Autodesk Fusion 360 part; units mm, degrees
sketch "Sketch1" plane through (0, 0, 0) normal (0, 0, 1) x (1, 0, 0)
  line L0 (0, 0) -> (60, 0)
  line L1 (60, 0) -> (60, 60)
  line L2 (60, 60) -> (0, 60)
  line L3 (0, 60) -> (0, 0)
  line L4 (5, 5) -> (55, 5)
  line L5 (55, 5) -> (55, 55)
  line L6 (55, 55) -> (5, 55)
  line L7 (5, 55) -> (5, 5)
  dimension "d1" = 60
  dimension "d2" = 60
extrude "Extrude1" add sketch "Sketch1" along normal blind 50
extrude "Extrude2" add sketch "Sketch1" along normal blind 43 contours L4 L5 L6 L7
sketch "Sketch2" plane through (0, 0, 43) normal (0, 0, 1) x (-1, 0, 0)
  line L0 (-5, -55) -> (-5, -5)
  line L1 (-5, -5) -> (-55, -5)
  line L2 (-55, -5) -> (-55, -55)
  line L3 (-55, -55) -> (-5, -55)
  circle A0 centre (-15, -45) radius 5
  circle A1 centre (-30, -45) radius 5
  circle A2 centre (-45, -45) radius 5
  circle A3 centre (-15, -30) radius 5
  circle A4 centre (-30, -30) radius 5
  circle A5 centre (-45, -30) radius 5
  circle A6 centre (-15, -15) radius 5
  circle A7 centre (-30, -15) radius 5
  circle A8 centre (-45, -15) radius 5
  dimension "d7" = 10
  dimension "d8" = 10
  dimension "d9" = 10
  dimension "d10" = 10
  dimension "d11" = 10
  dimension "d12" = 10
  dimension "d13" = 10
  dimension "d14" = 10
  dimension "d15" = 10
hole "Hole1" at (45, 45, 43) at (45, 30, 43) at (45, 15, 43) at (30, 15, 43) at (30, 30, 43) at (30, 45, 43) at (15, 45, 43) at (15, 30, 43) at (15, 15, 43) direction (0, 0, -1) diameter 10 depth 2 tip angle 15
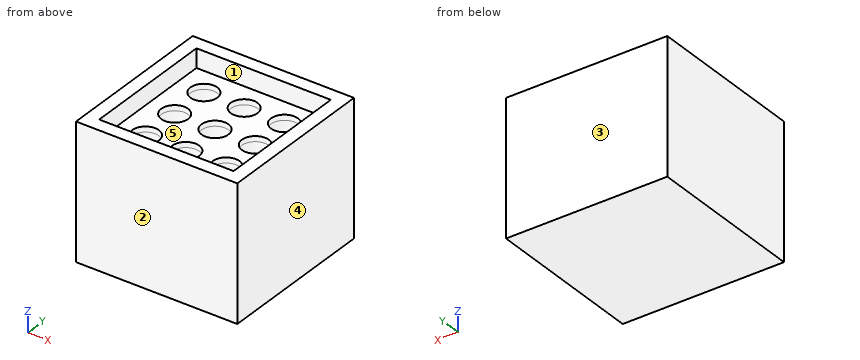
Geometry: final body of the model. Coordinates: model frame, mm. Face numbers are marked on the shaded views. A direction names the side the tool comes from. Round coordinates to 2 decimals unless told otherwise and drop trailing zeros. Loops run counter-clockwise (first coordinate to the right, second up) from the corner with the lowest first, then second, coordinate; pieces in that order, holes last. Notation, with made-up numbers: M 78,53.25 L 110,53.25 A14 ccw 110,70.25 Z; hole C -0.75,-1.5 d4. An arc over 180 degrees is marked long. Put each result on its own line as item: value. Start each with the question number.
(1) Set-up query: the marked faces 4 and 5. Return all of +Z, -Z, +X, -X, +Y, -Y with unobstructed straight access to the full face (end or side cutting, diameter ignored); none if empty.
(2) Section query B-B (x = 37). Return loops of the section in (y, z).
(3) Material intervals for line 1 along Y through (x, z) = (45, 42); line 2 along Y through (x, z) = (11, 46), sorted ascending. Write a range as [from, to].
(4) Contact query for a flat-ended pin moving along its axis: pin 1 Ø1 at (x, y) = (49, 6.5) entering from +Z. Output: stop coordinate, or through.
(5) Draft query along Y for the marked faces 1, 2 and 3. Return one class per face: +Y half, -Y half, draft (parallel to the pull), parting line (faces both ways), or undercut.
(6) Section query A-A (z = 26). State how many separate pieces and enclosed holes the cut face has, then the cut area to 3 significant figures.
Findings below:
1. face 4: +Z, -Z, +X, +Y, -Y
1. face 5: +Z
2. outline: M 0,0 L 60,0 L 60,50 L 55,50 L 55,43 L 5,43 L 5,50 L 0,50 Z
3. line 1: y = [0, 10], [20, 25], [35, 40], [50, 60]
3. line 2: y = [0, 5], [55, 60]
4. pin 1: stops at z = 43
5. face 1: undercut
5. face 2: -Y half
5. face 3: +Y half
6. separate pieces: 1
6. enclosed holes: 9
6. area: 3,340 mm2
